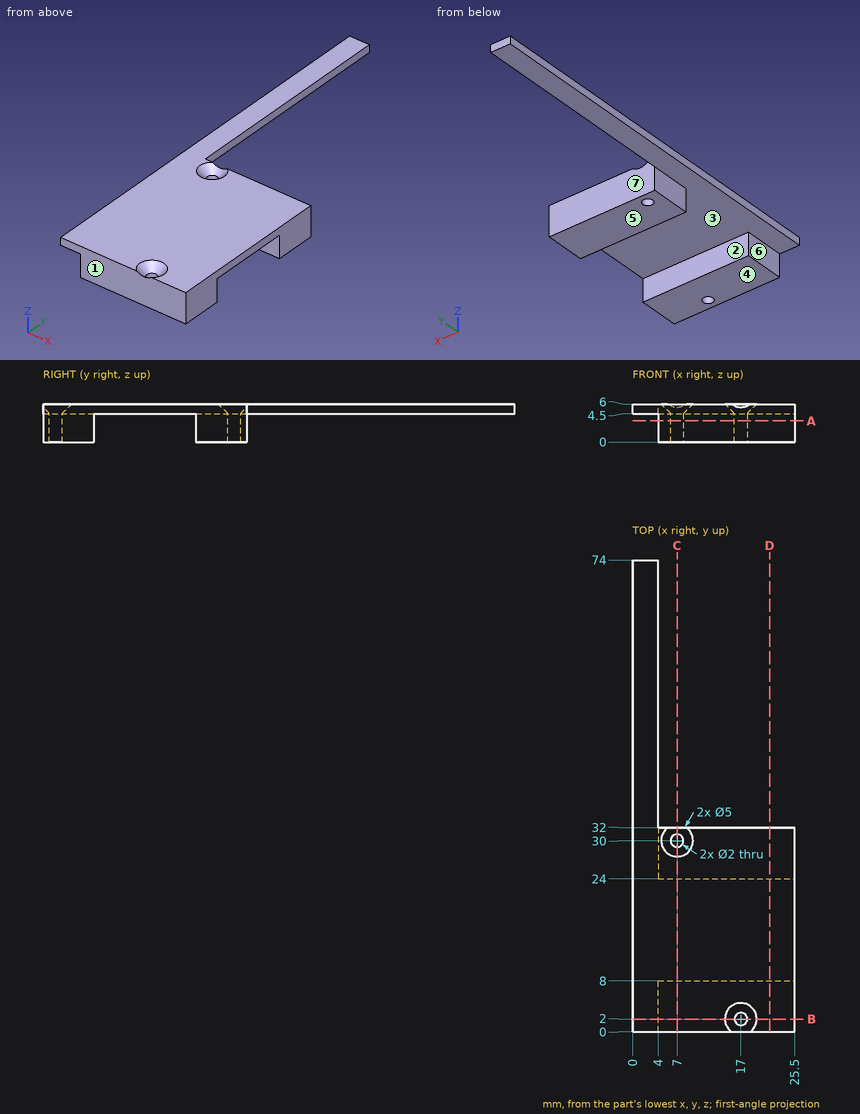
Study the drawing (mm; zero at the part's minimum x, y, z) and answer. A direction names the side the tool comes from. Coordinates: 2 decimals unless noted, no trailing zeros. Write each loop counter-clockwise with the first axis right and the second up, starting at its lowest first coordinate (ties: lowest second). Pieces come first, ordered by that corner, then holes. Notation, with made-up numbers: M -27,2 L -6,2 A17 cw -6,21 Z; hole C -27,-23.5 d8. An arc over 180 degrees is marked long. Use a Markdown table: item, result. Add a question column.
1. Section C-C (x = 7) is taken. Give the vertices of the cut face in (y, z).
2. Given P1, Ø0.8, axis at y = 54, z = 5, coming from the +X side; P2, Ø1.8, axis at x = 19, z = 3.5, coming from the +Y side; P3, Ø2, axis at y = 3.5, z = 1, coming from the -X side; P4, Ø2, axis at y = 38, z = 2, coming from the +X side, each flat-ended and moving along its own axis, determine where each tip first touches the part or whether it passes through.
3. Which of the six approach directions +Z, -Z, +X, -X, +Y, -Y give full straight-line access (tool end or side, diameter ignored) to the marked faces 5, 6 and 7?
4. Section D-D (x = 21.5) is taken. Give the vertices of the cut face in (y, z).
5. Straight lines are drawn through the part: line 1 along Y through (x, z) = (17, 1.2); line 2 along Y through (x, z) = (7, 2.8); line 3 along Y through (x, z) = (22.5, 0.4). For each, find the intervals that lie inside material, in ascending order. Write a range as [from, to].
6. For a pull along Y with two mould halves and no side action, classify the marked faces 1, 2, 3 and 4 as +Y half, -Y half, draft (parallel to the pull), parting line (faces both ways), or undercut.
7. Section B-B (y = 2) is taken. Give the vertices of the cut face in (x, z).
8. Section A-A (z = 3.35) is taken. Give the vertices of the cut face in (x, y).
Data:
| question | item | result |
|---|---|---|
| 1 | outline | M 0,0 L 8,0 L 8,4.5 L 24,4.5 L 24,0 L 29,0 L 29,4.5 L 27.5,6 L 0,6 Z; M 31,0 L 32,0 L 32,5.5 L 31,4.5 Z |
| 2 | P1 | stops at x = 4 |
| 2 | P2 | stops at y = 32 |
| 2 | P3 | stops at x = 4 |
| 2 | P4 | passes through |
| 3 | face 5 | -Z, +X, -X, +Y, -Y |
| 3 | face 6 | -Z, -X, +Y, -Y |
| 3 | face 7 | +Z, -Z, +X, +Y |
| 4 | outline | M 0,0 L 8,0 L 8,4.5 L 24,4.5 L 24,0 L 32,0 L 32,6 L 0,6 Z |
| 5 | line 1 | y = [0, 1], [3, 8], [24, 32] |
| 5 | line 2 | y = [0, 8], [24, 29], [31, 32] |
| 5 | line 3 | y = [0, 8], [24, 32] |
| 6 | face 1 | -Y half |
| 6 | face 2 | undercut |
| 6 | face 3 | undercut |
| 6 | face 4 | draft |
| 7 | outline | M 0,4.5 L 4,4.5 L 4,0 L 16,0 L 16,4.5 L 14.5,6 L 0,6 Z; M 18,0 L 25.5,0 L 25.5,6 L 19.5,6 L 18,4.5 Z |
| 8 | outline | M 4,0 L 25.5,0 L 25.5,8 L 4,8 Z; M 4,24 L 25.5,24 L 25.5,32 L 4,32 Z; hole C 7,30 d2; hole C 17,2 d2 |
